Read the model definition and answer for the solid it produces. Units are mm, in the model's axes. A direction names the side the tool comes from. Coordinates: 2 decimals unless noted, no trailing zeros. Order: outer loops, then holes, each group sorted by start corner. A loop starts at its lowest first (then second) coordinate and runs counter-clockwise, first axis right, second up. Notation, with made-up numbers: M 78.25,67.25 L 110.25,67.25 A29 ccw 110.25,104.25 Z; hole C 14,53 d9. An arc over 180 degrees is marked long. Put each result on its own line as item: value.
from build123d import *

# Parameters (mm, degrees)
F0_W     = 65.8
F0_H     = 98.8
F1_DEPTH = 35
F2_R     = 25
F4_DEPTH = 33
F6_DEPTH = 65.801
F7_R     = 5
F8_R     = 5
F9_R     = 6


with BuildPart() as f1:
    # F0 (on Top) → F1 (new body)
    with BuildSketch(Plane.XY):
        Rectangle(F0_W, F0_H)
    extrude(amount=F1_DEPTH)

    # F2
    f2_edges = [f1.edges().sort_by_distance(p)[0] for p in [
        (32.9, 49.4, 17.5),
        (-32.9, 49.4, 17.5),
        (32.9, -49.4, 17.5),
        (-32.9, -49.4, 17.5),
    ]]
    fillet(f2_edges, radius=F2_R)

    # F3 (on face) → F4 (cut)
    with BuildSketch(Plane.XY.offset(35)):
        with BuildLine():
            Line((31.4, -24.4), (31.4, 24.4))
            ThreePointArc((31.4, 24.4), (24.5170093579, 41.0170093579), (7.9, 47.9))
            Line((7.9, 47.9), (-7.9, 47.9))
            ThreePointArc((-7.9, 47.9), (-24.5170093579, 41.0170093579), (-31.4, 24.4))
            Line((-31.4, 24.4), (-31.4, -24.4))
            ThreePointArc((-31.4, -24.4), (-24.5170093579, -41.0170093579), (-7.9, -47.9))
            Line((-7.9, -47.9), (7.9, -47.9))
            ThreePointArc((7.9, -47.9), (24.5170093579, -41.0170093579), (31.4, -24.4))
        make_face()
    extrude(amount=-F4_DEPTH, mode=Mode.SUBTRACT)

    # F5 (on face) → F6 (cut, through all)
    with BuildSketch(Plane.YZ.offset(32.9)):
        with BuildLine():
            ThreePointArc((-12.5715859231, 35), (0, 22.4284140769), (12.5715859231, 35))
            Line((12.5715859231, 35), (-12.5715859231, 35))
        make_face()
    extrude(amount=-F6_DEPTH, mode=Mode.SUBTRACT)

    # F7
    f7_edges = [f1.edges().sort_by_distance(p)[0] for p in [
        (32.15, 12.571586, 35),
        (-32.15, 12.571586, 35),
        (32.15, -12.571586, 35),
        (-32.15, -12.571586, 35),
    ]]
    fillet(f7_edges, radius=F7_R)

    # F8
    f8_edges = [f1.edges().sort_by_distance(p)[0] for p in [
        (-24.517009, 41.017009, 2),
    ]]
    fillet(f8_edges, radius=F8_R)

    # F9
    f9_edges = [f1.edges().sort_by_distance(p)[0] for p in [
        (-25.57767, -42.07767, 0),
    ]]
    fillet(f9_edges, radius=F9_R)


solid = f1.part
Q1. A tool of negligible diameter and unlimited length cuts with its end or side. For faces 5 (the face through (-25.771, -41.882, 20.703)), 6 (the face through (32.14, 13.891, 34.034)), 7 (the face through (-0.11, 46.47, 3.5)), from which of +Z, -Z, +X, -X, +Y, -Y can it reach the whole face along a straight path? Write none if from no direction.
Answers below:
face 5: +Z, -Z, -X, -Y
face 6: +Z, +X, -X
face 7: +Z
Q2. Find section A-A on z = 32.5. Write down the section's boundary in (x, y).
Answers below:
outline: M -32.9,-24.4 A25 ccw -7.9,-49.4 L 7.9,-49.4 A25 ccw 32.9,-24.4 L 32.9,-12.52 L 31.4,-12.52 L 31.4,-24.4 A23.5 cw 7.9,-47.9 L -7.9,-47.9 A23.5 cw -31.4,-24.4 L -31.4,-12.52 L -32.9,-12.52 Z; M -32.9,12.52 L -31.4,12.52 L -31.4,24.4 A23.5 cw -7.9,47.9 L 7.9,47.9 A23.5 cw 31.4,24.4 L 31.4,12.52 L 32.9,12.52 L 32.9,24.4 A25 ccw 7.9,49.4 L -7.9,49.4 A25 ccw -32.9,24.4 Z
Q3. Find section C-C on x = 2. Write down the section's boundary in (y, z).
Answers below:
outline: M -49.4,6 A6 ccw -43.4,0 L 43.4,0 A6 ccw 49.4,6 L 49.4,35 L 47.9,35 L 47.9,7 A5 cw 42.9,2 L -42.9,2 A5 cw -47.9,7 L -47.9,35 L -49.4,35 Z
Q4. Given pin 1 (6 mm diameter, centred on x = 21, y = -38.5, fed in from -Z); pin 2 (1 mm diameter, centred on x = 4.5, y = 38.5, fed in from +Z); pin 3 (5 mm diameter, centred on x = 23, z = 12.5, fed in from +Y); pin 4 (5 mm diameter, centred on x = -19.5, z = 22, fed in from -Y) (3 decimals), each flat-ended and moving along its own axis, determine where each tip first touches the part or whether it passes through.
Answers below:
pin 1: stops at z = 0
pin 2: stops at z = 2
pin 3: stops at y = 45.99
pin 4: stops at y = -47.685
Q5. For a pull along Y with two mould halves and no side action, classify faces 1 (the face through (25.771, 41.882, 20.703)), 2 (the face through (0, 47.9, 21)), 3 (the face through (-32.9, 0, 17)), 4 (the face through (24.7, 40.83, 21.2)) as +Y half, -Y half, draft (parallel to the pull), parting line (faces both ways), or undercut.
Answers below:
face 1: +Y half
face 2: undercut
face 3: draft
face 4: undercut
Q6. Find section B-B on z = 19. Write down the section's boundary in (x, y).
Answers below:
outline: M -32.9,-24.4 A25 ccw -7.9,-49.4 L 7.9,-49.4 A25 ccw 32.9,-24.4 L 32.9,24.4 A25 ccw 7.9,49.4 L -7.9,49.4 A25 ccw -32.9,24.4 Z; hole M -31.4,-24.4 A23.5 ccw -7.9,-47.9 L 7.9,-47.9 A23.5 ccw 31.4,-24.4 L 31.4,24.4 A23.5 ccw 7.9,47.9 L -7.9,47.9 A23.5 ccw -31.4,24.4 Z
Q7. Find section D-D on y = -15.5. Write down the section's boundary in (x, z).
Answers below:
outline: M -32.9,6 A6 ccw -26.9,0 L 26.9,0 A6 ccw 32.9,6 L 32.9,34.82 L 31.4,34.82 L 31.4,7 A5 cw 26.4,2 L -26.4,2 A5 cw -31.4,7 L -31.4,34.82 L -32.9,34.82 Z
Q8. Consider line 1 along X through (y, z) = (8.5, 20.5); line 2 along Y through (x, z) = (-8.5, 29); line 3 along X through (y, z) = (-43, 18.5). Determine where each line is inside the solid, lowest interval first.
Answers below:
line 1: x = -32.9 to -31.4, 31.4 to 32.9
line 2: y = -49.39 to -47.89, 47.89 to 49.39
line 3: x = -24.6 to -22.26, 22.26 to 24.6
